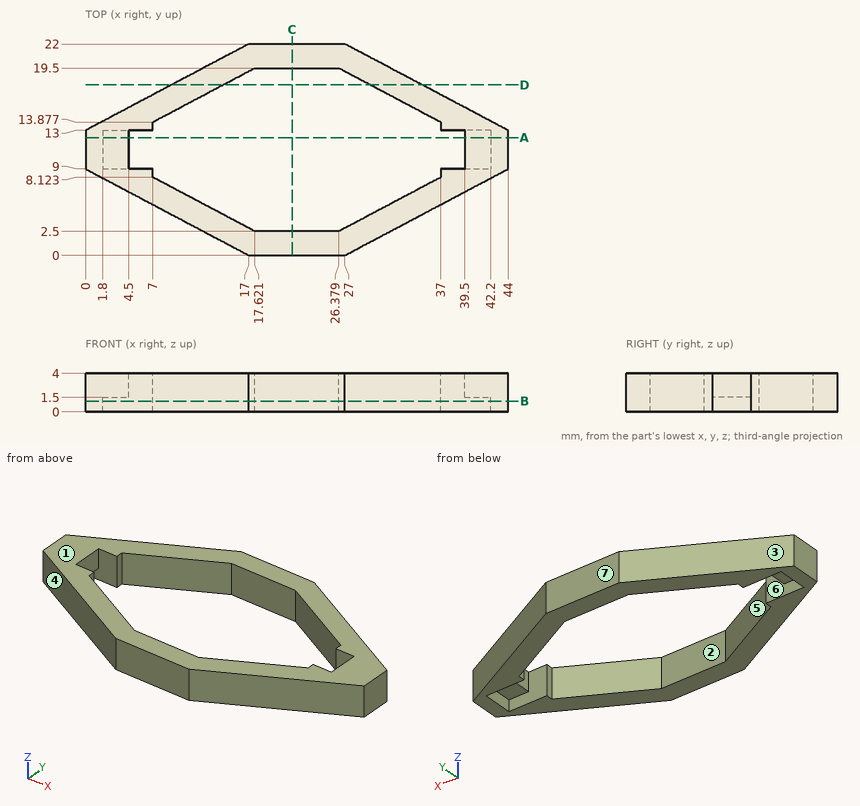
For this review, use the dimensioned drawing (mm, ordinates from the lowest corner) and the shaded views. A direction names the side the tool comes from. Give positions to 0.01 mm unless a question says otherwise; leave off trailing zeros. Order: outer loops, then holes, each group sorted by start corner. A loop starts at its lowest first (then second) coordinate and runs counter-clockwise, first axis right, second up. Notation, with made-up numbers: M -22.75,19.25 L 24.25,19.25 A17 cw 24.25,33.25 Z; hole C 54,0 d4. An arc over 180 degrees is marked long. Use one line per item in the form item = value. Start each with the question number.
Item 1: To check wall thickness, follow line 1 along X through (y, z) = (10, 2.2); line 2 along Y through (x, z) = (26, 3.5); line 3 along Y through (x, z) = (11, 2.8) (1 decimal). State the ranges of each line that lie inside material, in increasing order. Write a range as from..to.
Item 2: We need section A-A on y = 12.25. Give the boundary of the cut face in (x, z), plus the area to 3 significant figures.
Item 3: Insertion check: pin 1 Ø1 at (x, y) = (25.5, 17.5) entering from -Z; pin 2 Ø1.4 at (x, y) = (40.5, 10.5) entering from -Z; pin 3 Ø1 at (x, z) = (14.5, 1.5) entering from -Y; pin 4 Ø1.2 at (x, z) = (5, 2.5) entering from -Y (1 decimal). Each pin has a flat end and moves straight along its axis. Give the tip position at first contact, or say it passes through.
Item 4: We need section B-B on z = 1.1. Give the boundary of the cut face in (x, y).
Item 5: For the marked faces 5, 6 and 7, list the 3-axis set-ups (+Z, -Z, +X, -X, +Y, -Y) from which the entire face can be reached by the end or side of a thin tool; tool diameter is ignored.
Item 6: The part is to be moulded in two halves that separate along Y. For the marked faces 1, 2, 3 and 4, say which applies: pulls with the +Y half, pulls with the -Y half, needs draft (parallel to the pull), parting line crosses it, or undercut.
Item 7: We need section D-D on y = 17.75. Give the boundary of the cut face in (x, z).
Item 8: We need section C-C on x = 21.5. Give the boundary of the cut face in (y, z).
Completed:
q1.line_1 = 0..4.5, 39.5..44
q1.line_2 = 0..2.5, 19.5..22
q1.line_3 = 3.2..6, 16..18.8
q2.outline = M 0,0 L 1.8,0 L 1.8,1.5 L 4.5,1.5 L 4.5,4 L 0,4 Z; M 39.5,1.5 L 42.2,1.5 L 42.2,0 L 44,0 L 44,4 L 39.5,4 Z
q2.area = 27.9 mm²
q3.pin_1 = through
q3.pin_2 = 1.5
q3.pin_3 = 1.06
q3.pin_4 = 6
q4.outline = M 0,9 L 17,0 L 27,0 L 44,9 L 44,13 L 27,22 L 17,22 L 0,13 Z; hole M 1.8,9 L 7,9 L 7,8.12 L 17.62,2.5 L 26.38,2.5 L 37,8.12 L 37,9 L 42.2,9 L 42.2,13 L 37,13 L 37,13.88 L 26.38,19.5 L 17.62,19.5 L 7,13.88 L 7,13 L 1.8,13 Z
q5.face_5 = +Z, -Z
q5.face_6 = -Z
q5.face_7 = +Z, -Z, +X, -X, +Y
q6.face_1 = needs draft
q6.face_2 = undercut
q6.face_3 = pulls with the +Y half
q6.face_4 = pulls with the -Y half
q7.outline = M 8.97,0 L 14.32,0 L 14.32,4 L 8.97,4 Z; M 29.68,0 L 35.03,0 L 35.03,4 L 29.68,4 Z
q8.outline = M 0,0 L 2.5,0 L 2.5,4 L 0,4 Z; M 19.5,0 L 22,0 L 22,4 L 19.5,4 Z
